```python
from build123d import *

# Parameters (mm, degrees)
SKETCH_1_W          = 85
SKETCH_1_H          = 5
SKETCH_2_R          = 12.5
SKETCH_2_R_2        = 7.5
SKETCH_2_R_3        = 3
CUT_EXTRUDE_1_DEPTH = 20


with BuildPart() as part:
    # 草图1 → 旋转1 (revolve)
    with BuildSketch(Plane.XY):
        with Locations((-42.5, 2.5)):
            Rectangle(SKETCH_1_W, SKETCH_1_H)
    revolve(axis=Axis((0, 0, 0), (0, 1, 0)))

    # 草图2 → 切除-拉伸1 (cut)
    with BuildSketch(Plane(origin=(0, 0, 0), x_dir=(1, 0, 0), z_dir=(0, 1, 0))):
        with Locations((50, 0)):
            Circle(SKETCH_2_R)
        Circle(SKETCH_2_R_2)
        with Locations((-50, 0)):
            Circle(SKETCH_2_R_3)
        with Locations((25, 43.301270189)):
            Circle(SKETCH_2_R_3)
        with Locations((25, -43.301270189)):
            Circle(SKETCH_2_R_3)
    extrude(amount=CUT_EXTRUDE_1_DEPTH, mode=Mode.SUBTRACT)


solid = part.part
```
The model under review builds one solid part; all positions refer to its coordinate system, in mm. Round coordinates to 2 decimals unless told otherwise and drop trailing zeros. Loops run counter-clockwise (first coordinate to the right, second up) from the corner with the lowest first, then second, coordinate; pieces in that order, holes last. Notation, with made-up numbers: M -28,-36 L -6,-36 A13 ccw -6,-30 Z; hole C -28.5,79.25 d9. An arc over 180 degrees is marked long. Answer as a JSON object with one key per item and string values.
(1) Take a section at C-C on x = 25. Give the boundary of the cut face in (y, z).
Resolved:
{"outline": "M 0,-81.24 L 5,-81.24 L 5,-46.3 L 0,-46.3 Z; M 0,-40.3 L 5,-40.3 L 5,40.3 L 0,40.3 Z; M 0,46.3 L 5,46.3 L 5,81.24 L 0,81.24 Z"}
(2) Take a section at B-B on z = 5. Give the boundary of the cut face in (x, y).
Resolved:
{"outline": "M -84.85,0 L -5.59,0 L -5.59,5 L -84.85,5 Z; M 5.59,0 L 38.54,0 L 38.54,5 L 5.59,5 Z; M 61.46,0 L 84.85,0 L 84.85,5 L 61.46,5 Z"}
(3) Take a section at D-D on x = -50. Give the boundary of the cut face in (y, z), and give its area (3 significant figures).
Resolved:
{"outline": "M 0,-68.74 L 5,-68.74 L 5,-3 L 0,-3 Z; M 0,3 L 5,3 L 5,68.74 L 0,68.74 Z", "area": "657 mm²"}
(4) To check wall thickness, follow line 1 along Z through (x, y) = (0, 1.8); line 2 along Z through (x, y) = (25, 3.85); line 3 along Z through (x, y) = (44, 0.35). State the ranges of each line that lie inside material, in increasing order.
Resolved:
{"line 1": "-85 to -7.5, 7.5 to 85", "line 2": "-81.24 to -46.3, -40.3 to 40.3, 46.3 to 81.24", "line 3": "-72.73 to -10.97, 10.97 to 72.73"}
(5) Take a section at A-A on x = 0. Give the boundary of the cut face in (y, z), and give its area (3 significant figures).
Resolved:
{"outline": "M 0,-85 L 5,-85 L 5,-7.5 L 0,-7.5 Z; M 0,7.5 L 5,7.5 L 5,85 L 0,85 Z", "area": "775 mm²"}
(6) Draft analysis for pull direction Z (two halves, no side actions). For faces 1 (the cylindrical face through (67.453, 2.535, -51.721)), 2 (the cylindrical face through (24.35, 2.46, 46.23)), 3 (the cylindrical face through (-7.493, 2.465, -0.33)), 4 (the flat face through (-18, 5, 1)), state which applies: released by +Z, released by -Z, zero draft, split by the parting line, or undercut.
Resolved:
{"face 1": "split by the parting line", "face 2": "undercut", "face 3": "undercut", "face 4": "zero draft"}
(7) Clearance check with flat-ended pins moving along their axes: P1, Ø13.5, axis at x = 0, z = 0, coming from the -Y side (3 decimals); P2, Ø2, axis at x = -48, y = 1.5, coming from the +Z side; P3, Ø1.5, axis at y = 2.5, z = 42.5, coming from the +X side. State where each tip first meets the part, or that it passes through.
Resolved:
{"P1": "through", "P2": "z = 70.82", "P3": "x = 74.04"}
